Input: part model. Units: mm. Frame: model coordinates. Give positions to 0.01 mm unless a question says otherwise; leave off trailing zeros. Loops run counter-clockwise (first coordinate to the right, second up) from the corner with the lowest first, then second, coordinate; pieces in that order, holes last. Notation, with made-up numbers: (75, -7) -> (96, -7) arc R37 ccw to (96, 29) -> close; hole circle Ø7 at (72.5, -21). An arc over 180 degrees is marked (long way). Answer as a JSON object with one key per item and string values.
Autodesk Inventor part; units mm, degrees
ref_plane "YZ Plane" through (0, 0, 0) normal (1, 0, 0) x (0, 1, 0)
ref_plane "XZ Plane" through (0, 0, 0) normal (0, 1, 0) x (-1, 0, 0)
ref_plane "XY Plane" through (0, 0, 0) normal (0, 0, 1) x (1, 0, 0)
sketch "maiin" plane through (0, 0, 0) normal (0, 0, 1) x (1, 0, 0)
  arc A0 (6.5899, -1.511) -> (-1.5658, -0.8125) centre (2.0978, -5.9991) ccw
  circle A1 centre (-6.5018, 3.4753) radius 2.1844
  line L0 (-31.2537, -6.2516) -> (11.7059, 28.671)
  line L1 (-23.5847, -16.3655) -> (-1.5658, -0.8125)
  circle A2 centre (-27.2482, -11.1789) radius 2.1844
  arc A3 (-31.2537, -6.2516) -> (-23.5847, -16.3655) centre (-27.2482, -11.1789) ccw
  circle A4 centre (28.4, -14.3563) radius 2.1844
  line L2 (34.75, -14.3563) -> (34.75, 23.7437)
  line L3 (15.7114, 30.0937) -> (28.4, 30.0937)
  circle A5 centre (28.4, 23.7437) radius 2.1844
  circle A6 centre (28.4, -1.6563) radius 2.1844
  arc A7 (23.9079, -18.8444) -> (34.75, -14.3563) centre (28.4, -14.3563) ccw
  line L4 (23.9079, -18.8444) -> (6.5899, -1.511)
  circle A8 centre (15.7114, 23.7437) radius 2.1844
  circle A9 centre (15.7114, -1.6563) radius 2.1844
  arc A10 (34.75, 23.7437) -> (28.4, 30.0937) centre (28.4, 23.7437) ccw
  arc A11 (15.7114, 30.0937) -> (11.7059, 28.671) centre (15.7114, 23.7437) ccw
  point P0 (10.0881, 4.3711)
  dimension "d0" = 12.7
  dimension "d1" = 12.7
  dimension "d4" = 6.35
  dimension "d6" = 4.3688
sketch "Sketch1" plane through (0, 0, 0) normal (1, 0, 0) x (0, 1, 0)
  arc A0 (-21.8101, -25.2546) -> (-29.9658, -24.5561) centre (-26.3022, -29.7428) ccw
  circle A1 centre (-34.9019, -20.2684) radius 2.1844
  line L0 (-59.6538, -29.9953) -> (-16.6941, 4.9273)
  line L1 (-51.9847, -40.1092) -> (-29.9658, -24.5561)
  circle A2 centre (-55.6483, -34.9226) radius 2.1844
  arc A3 (-59.6538, -29.9953) -> (-51.9847, -40.1092) centre (-55.6483, -34.9226) ccw
  circle A4 centre (0, -38.1) radius 2.1844
  line L2 (6.35, -38.1) -> (6.35, 0)
  line L3 (-12.6886, 6.35) -> (0, 6.35)
  circle A5 centre (0, 0) radius 2.1844
  circle A6 centre (0, -25.4) radius 2.1844
  arc A7 (-4.4921, -42.5881) -> (6.35, -38.1) centre (0, -38.1) ccw
  line L4 (-4.4921, -42.5881) -> (-21.8101, -25.2546)
  circle A8 centre (-12.6886, 0) radius 2.1844
  circle A9 centre (-12.6886, -25.4) radius 2.1844
  arc A10 (6.35, 0) -> (0, 6.35) centre (0, 0) ccw
  arc A11 (-12.6886, 6.35) -> (-16.6941, 4.9273) centre (-12.6886, 0) ccw
extrude "Extrusion1" add sketch "Sketch1" along normal blind 1.5875
properties part number "triangle_brace_gusset"
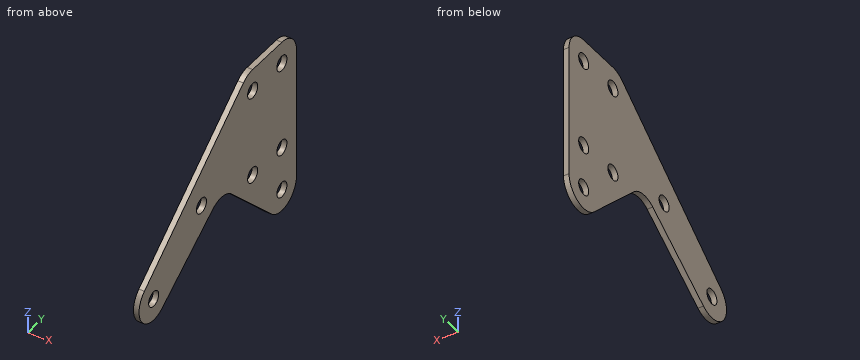
Q1. Section B-B, the plane x = 1.1. Return the cut outline in (y, z), then the cut area to 3 significant figures.
Evaluation:
{"outline": "(-59.65, -30) arc R6.35 ccw to (-51.98, -40.11) -> (-29.97, -24.56) arc R6.35 cw to (-21.81, -25.25) -> (-4.49, -42.59) arc R6.35 ccw to (6.35, -38.1) -> (6.35, 0) arc R6.35 ccw to (0, 6.35) -> (-12.69, 6.35) arc R6.35 ccw to (-16.69, 4.93) -> close; hole circle Ø4.37 at (-55.65, -34.92); hole circle Ø4.37 at (-34.9, -20.27); hole circle Ø4.37 at (-12.69, -25.4); hole circle Ø4.37 at (-12.69, 0); hole circle Ø4.37 at (0, -38.1); hole circle Ø4.37 at (0, -25.4); hole circle Ø4.37 at (0, 0)", "area": "1,790 mm2"}
Q2. Section D-D, the plane y = -9. Return the cut outline in (x, z).
Evaluation:
{"outline": "(0, -38.08) -> (1.59, -38.08) -> (1.59, 6.35) -> (0, 6.35) -> close"}
Q3. Ray query, line 1 along Z through (x, y) = (1, 0); line 2 along Y through (x, z) = (0.55, -25.5); line 3 along Y through (x, z) = (0.3, -39). Return the intervals inside material, ascending.
Evaluation:
{"line 1": "z = -44.45 to -40.28, -35.92 to -27.58, -23.22 to -2.18, 2.18 to 6.35", "line 2": "y = -54.12 to -31.3, -21.56 to -14.87, -10.51 to -2.18, 2.18 to 6.35", "line 3": "y = -60.52 to -50.41, -8.08 to -1.99, 1.99 to 6.29"}
Q4. Section C-C, the plane z = 3.5. Return the cut outline in (x, y), then the cut area to 3 significant figures.
Evaluation:
{"outline": "(0, -18.45) -> (1.59, -18.45) -> (1.59, 5.3) -> (0, 5.3) -> close", "area": "37.7 mm2"}
Q5. Pin query (flat end, axial travel): pin 1 (6 mm diameter, centred on y = -14.5, z = -39, fed in from -X). Return the tip coordinate at first contact, or that it passes through.
Evaluation:
{"pin 1": "passes through"}
Q6. Section A-A, the plane y = -57. Return the cut outline in (x, z).
Evaluation:
{"outline": "(0, -41.13) -> (1.59, -41.13) -> (1.59, -36.64) -> (0, -36.64) -> close; (0, -33.21) -> (1.59, -33.21) -> (1.59, -27.84) -> (0, -27.84) -> close"}
